```python
from build123d import *

# Parameters (mm, degrees)
SKETCH1_W           = 76.2
SKETCH1_H           = 63.5
BOSS_EXTRUDE1_DEPTH = 2.54
SKETCH2_W           = 76.2
SKETCH2_H           = 6.75
BOSS_EXTRUDE2_DEPTH = 4
SKETCH3_R           = 2.032
CUT_EXTRUDE1_DEPTH  = 3.81
SKETCH4_R           = 15
CUT_EXTRUDE2_DEPTH  = 10
SKETCH5_W           = 3.81
SKETCH5_H           = 10.16
BOSS_EXTRUDE3_DEPTH = 1.27


with BuildPart() as part:
    # Sketch1 → Boss-Extrude1 (new body)
    with BuildSketch(Plane.XY):
        with Locations((38.1, 31.75)):
            Rectangle(SKETCH1_W, SKETCH1_H)
    extrude(amount=BOSS_EXTRUDE1_DEPTH)

    # Sketch2 → Boss-Extrude2 (add)
    with BuildSketch(Plane(origin=(0, 0, 0), x_dir=(-1, 0, 0), z_dir=(0, 0, -1))):
        with Locations((-38.1, 60.125)):
            Rectangle(SKETCH2_W, SKETCH2_H)
        with Locations((-38.1, 3.375)):
            Rectangle(SKETCH2_W, SKETCH2_H)
    extrude(amount=BOSS_EXTRUDE2_DEPTH)

    # Sketch3 → Cut-Extrude1 (cut)
    with BuildSketch(Plane(origin=(0, 0, -4), x_dir=(-1, 0, 0), z_dir=(0, 0, -1))):
        with Locations((-63.5, 60.125)):
            Circle(SKETCH3_R)
        with Locations((-63.5, 3.375)):
            Circle(SKETCH3_R)
        with Locations((-12.7, 3.375)):
            Circle(SKETCH3_R)
        with Locations((-12.7, 60.125)):
            Circle(SKETCH3_R)
    extrude(amount=-CUT_EXTRUDE1_DEPTH, mode=Mode.SUBTRACT)

    # Sketch4 → Cut-Extrude2 (cut)
    with BuildSketch(Plane.XY.offset(2.54)):
        with Locations((38.1, 31.75)):
            Circle(SKETCH4_R)
    extrude(amount=-CUT_EXTRUDE2_DEPTH, mode=Mode.SUBTRACT)

    # Sketch5 → Boss-Extrude3 (add)
    with BuildSketch(Plane(origin=(0, 0, 0), x_dir=(-1, 0, 0), z_dir=(0, 0, -1))):
        with Locations((-26.035, 51.67)):
            Rectangle(SKETCH5_W, SKETCH5_H)
        with Locations((-26.035, 11.83)):
            Rectangle(SKETCH5_W, SKETCH5_H)
    extrude(amount=BOSS_EXTRUDE3_DEPTH)


solid = part.part
```
Design review of the part built by this model. Coordinates are the model's own, in mm. A direction names the side the tool comes from. Give positions to 0.01 mm unless a question says otherwise; leave off trailing zeros. Write each loop counter-clockwise with the first axis right and the second up, starting at its lowest first coordinate (ties: lowest second). Pieces come first, ordered by that corner, then holes.
(1) Wall thickness on line 1 along Y through (x, z) = (12.7, -1.6); line 2 along Y through (x, z) = (53, -0.75); line 3 along X through (y, z) = (31, 1.5): over which ranges is each line inside the solid? List them lowest first.
Checked values:
line 1: y = 0 to 1.34, 5.41 to 6.75, 56.75 to 58.09, 62.16 to 63.5
line 2: y = 0 to 6.75, 56.75 to 63.5
line 3: x = 0 to 23.12, 53.08 to 76.2
(2) Add section A-A (x = 38.1). Give the boundary of the cut face in (y, z), and give its area (3 significant figures).
Checked values:
outline: (0, -4) - (6.75, -4) - (6.75, 0) - (16.75, 0) - (16.75, 2.54) - (0, 2.54) - close; (46.75, 0) - (56.75, 0) - (56.75, -4) - (63.5, -4) - (63.5, 2.54) - (46.75, 2.54) - close
area: 139 mm2
(3) Clearance check with flat-ended pins moving along their axes: pin 1 Ø10 at (x, y) = (62, 42.5) entering from -Z; pin 2 Ø1.2 at (x, y) = (13.5, 60) entering from -Z; pin 3 Ø1.9 at (x, y) = (26, 50.5) entering from -Z. State where each tip first meets the part, or that it passes through.
Checked values:
pin 1: stops at z = 0
pin 2: stops at z = -0.19
pin 3: stops at z = -1.27
(4) Add section D-D (z = 1). Give the boundary of the cut face in (x, y), and give its area (3 significant figures).
Checked values:
outline: (0, 0) - (76.2, 0) - (76.2, 63.5) - (0, 63.5) - close; hole circle Ø30 at (38.1, 31.75)
area: 4,130 mm2
(5) Tool access review of faces 1 (the face through (64, 60, -0.19)), 2 (the face through (26, 12, -1.27)), 3 (the face through (39, 3, -4)): name each direction out of +Z, -Z, +X, -X, +Y, -Y from which nothing blocks a thin tool from reaching the whole face with its end or side.
Checked values:
face 1: -Z
face 2: -Z, +X, -X
face 3: -Z, +X, -X, +Y, -Y
(6) Mouldability with a two-part tool opening along Y and no side actions: class faces 4 (the face through (39, 56.75, -2)), 5 (the face through (46, 18, 2.54)), 6 (the face through (38, 0, -1)) as +Y half, -Y half, draft (parallel to the pull), parting line (faces both ways), or undercut.
Checked values:
face 4: undercut
face 5: draft
face 6: -Y half
(7) Add section C-C (z = -2.75). Give the boundary of the cut face in (x, y) (3 decimals).
Checked values:
outline: (0, 0) - (76.2, 0) - (76.2, 6.75) - (0, 6.75) - close; (0, 56.75) - (76.2, 56.75) - (76.2, 63.5) - (0, 63.5) - close; hole circle Ø4.064 at (12.7, 3.375); hole circle Ø4.064 at (12.7, 60.125); hole circle Ø4.064 at (63.5, 3.375); hole circle Ø4.064 at (63.5, 60.125)
(8) Add section B-B (y = 31.75). Give the boundary of the cut face in (x, z).
Checked values:
outline: (0, 0) - (23.1, 0) - (23.1, 2.54) - (0, 2.54) - close; (53.1, 0) - (76.2, 0) - (76.2, 2.54) - (53.1, 2.54) - close
